Build history of the part. All positions in model axes, mm. A direction names the side the tool comes from. Coordinates: 2 decimals unless noted, no trailing zeros. Write each loop counter-clockwise with the first axis right and the second up, starting at its lowest first coordinate (ties: lowest second). Pieces come first, ordered by that corner, then holes.
```python
from build123d import *

# Parameters (mm, degrees)
F1_DEPTH = 20.32
F3_DEPTH = 20.321
F5_DEPTH = 15.24


with BuildPart() as f1:
    # F0 (on Front) → F1 (new body)
    with BuildSketch(Plane.XZ):
        with BuildLine():
            Line((-25.4, 8.255), (-25.4, -12.7))
            Line((-25.4, -12.7), (25.4, -12.7))
            Line((25.4, -12.7), (25.4, 8.255))
            ThreePointArc((25.4, 8.255), (24.09809, 11.39809), (20.955, 12.7))
            Line((20.955, 12.7), (-20.955, 12.7))
            ThreePointArc((-20.955, 12.7), (-24.09809, 11.39809), (-25.4, 8.255))
        make_face()
    extrude(amount=F1_DEPTH)

    # F2 (on face) → F3 (cut, through all)
    with BuildSketch(Plane.XZ.offset(20.32)):
        with BuildLine():
            Line((9.525, 12.7), (-9.525, 12.7))
            ThreePointArc((-9.525, 12.7), (0, 3.175), (9.525, 12.7))
        make_face()
    extrude(amount=-F3_DEPTH, mode=Mode.SUBTRACT)

    # F4 (on face) → F5 (cut)
    with BuildSketch(Plane.XZ.offset(20.32)):
        with BuildLine():
            Line((-11.049, 5.08), (-11.049, 12.7))
            Line((-11.049, 12.7), (-20.955, 12.7))
            ThreePointArc((-20.955, 12.7), (-24.09809, 11.39809), (-25.4, 8.255))
            Line((-25.4, 8.255), (-25.4, -12.7))
            Line((-25.4, -12.7), (-20.955, -12.7))
            Line((-20.955, -12.7), (-20.955, 0))
            Line((-20.955, 0), (-16.129, 0))
            ThreePointArc((-16.129, 0), (-12.536898, 1.487898), (-11.049, 5.08))
        make_face()
        Polygon((-17.145, -12.7), (17.145, -12.7), (17.145, -5.715), (0, -5.715), (-17.145, -5.715), align=None)
        with BuildLine():
            Line((20.955, 12.7), (11.049, 12.7))
            Line((11.049, 12.7), (11.049, 5.08))
            ThreePointArc((11.049, 5.08), (12.536898, 1.487898), (16.129, 0))
            Line((16.129, 0), (20.955, 0))
            Line((20.955, 0), (20.955, -12.7))
            Line((20.955, -12.7), (25.4, -12.7))
            Line((25.4, -12.7), (25.4, 8.255))
            ThreePointArc((25.4, 8.255), (24.09809, 11.39809), (20.955, 12.7))
        make_face()
    extrude(amount=-F5_DEPTH, mode=Mode.SUBTRACT)


solid = f1.part
```
1. Saw through at C-C on x = 0. List the corners of the cut face in (y, z) (3 decimals), plus the area to 3 significant figures.
Computed values:
outline: (-20.32, -5.715) - (-5.08, -5.715) - (-5.08, -12.7) - (0, -12.7) - (0, 3.175) - (-20.32, 3.175) - close
area: 216 mm2
2. Saw through at D-D on z = 3.75. List the corners of the cut face in (x, y), plus the area to 3 significant figures.
Computed values:
outline: (-25.4, -5.08) - (-11.23, -5.08) - (-11.23, -20.32) - (-3.26, -20.32) - (-3.26, 0) - (-25.4, 0) - close; (3.26, -20.32) - (11.23, -20.32) - (11.23, -5.08) - (25.4, -5.08) - (25.4, 0) - (3.26, 0) - close
area: 468 mm2
3. Flat gauge pins, fed straight in: pin 1 (8.5 mm diameter, centred on y = -11.5, z = 8, fed in from -X); pin 2 (2 mm diameter, centred on x = 0.5, y = -11, fed in from +Z); pin 3 (1 mm diameter, centred on y = -15, z = 3.5, fed in from -X). Where does each tip first touch, or does it go through?
Computed values:
pin 1: stops at x = -11.23
pin 2: stops at z = 3.29
pin 3: stops at x = -11.49
4. 3-axis set-ups, long thin cutter, end or side, ignore diameter. For faces 1 (the face through (17.145, -13, -9)), 2 (the face through (-20.955, -13, -6)), 3 (the face through (19, -13, 0)), 4 (the face through (-19, -13, 0)): which of +Z, -Z, +X, -X, +Y, -Y reach the whole face in a straight line?
Computed values:
face 1: -Z, -Y
face 2: +Z, -Z, -X, -Y
face 3: +Z, +X, -Y
face 4: +Z, -X, -Y
5. Saw through at B-B on z = -4.75. List the corners of the cut face in (x, y) (3 decimals).
Computed values:
outline: (-25.4, -5.08) - (-20.955, -5.08) - (-20.955, -20.32) - (20.955, -20.32) - (20.955, -5.08) - (25.4, -5.08) - (25.4, 0) - (-25.4, 0) - close
6. Saw through at A-A on y = -3.75. List the corners of the cut face in (x, z) (3 decimals), plus the area to 3 significant figures.
Computed values:
outline: (-25.4, -12.7) - (25.4, -12.7) - (25.4, 8.255) arc R4.445 ccw to (20.955, 12.7) - (9.525, 12.7) arc R9.525 cw to (-9.525, 12.7) - (-20.955, 12.7) arc R4.445 ccw to (-25.4, 8.255) - close
area: 1,140 mm2
7. Mould opens along X. For faces 5 (the face through (0, -5.08, -9)), 6 (the face through (0, 0, 0)), 7 (the face through (-12.577, -12.807, 1.449)) say: +X half, -X half, draft (parallel to the pull), parting line (faces both ways), or undercut.
Computed values:
face 5: undercut
face 6: draft
face 7: -X half
8. Probe line 1 along X through (y, z) = (-13, -9.25) (3 decimals); line 2 along Z through (x, y) = (-18, -7.25); line 3 along X through (y, z) = (-17.25, -3.75) (3 decimals). List the from-to ranges inside material, lowest first.
Computed values:
line 1: x = -20.955 to -17.145, 17.145 to 20.955
line 2: z = -12.7 to 0
line 3: x = -20.955 to 20.955
